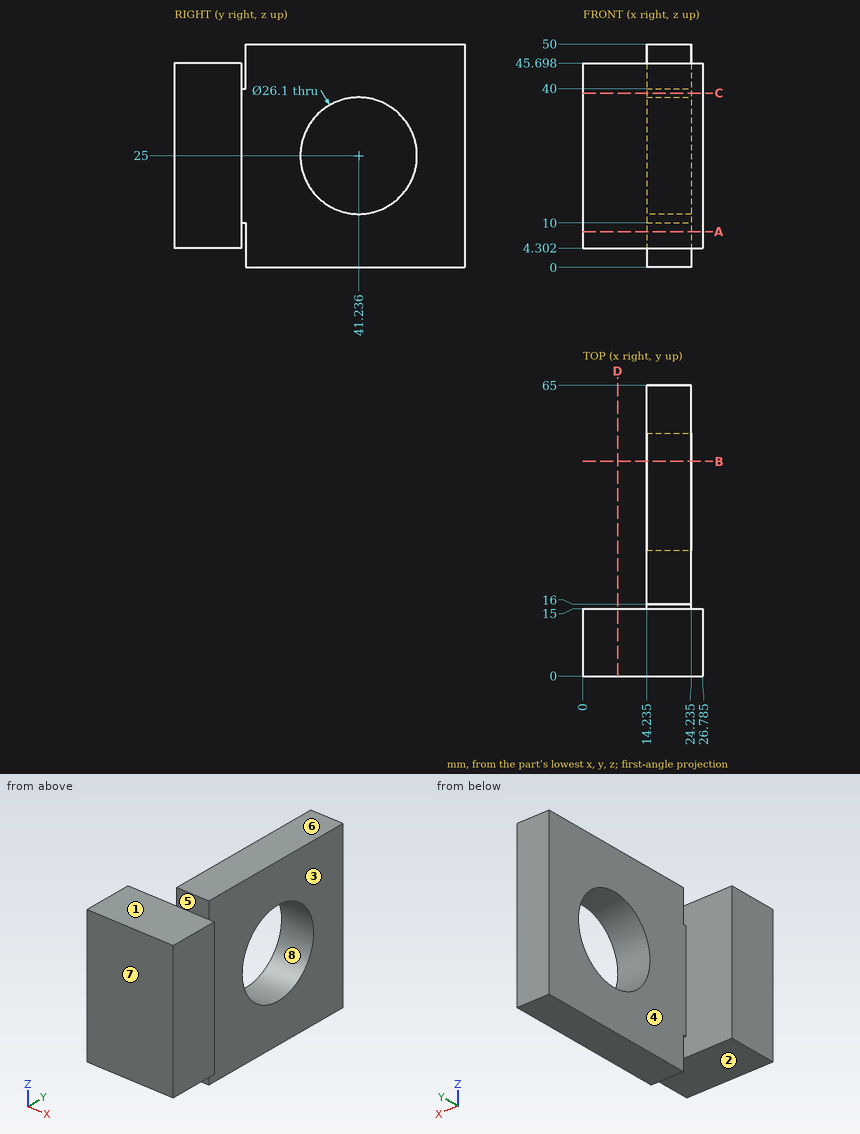
Design review of the part shown in the three views and the two pictorial views. Dimensions are in mm from the part's minimum x, y and z. A direction names the side the tool comes from. Round coordinates to 2 decimals unless told otherwise and drop trailing zeros. Write each loop counter-clockwise with the first axis right and the second up, starting at its lowest first coordinate (ties: lowest second). Pieces come first, ordered by that corner, then holes. Notation, with made-up numbers: (80, -3) - (132, -3) arc R21 cw to (132, 22) - close; hole circle Ø8 at (64, 82.25). An arc over 180 degrees is marked (long way). Return JSON: item names as keys, results as strings. Group by question number.
Item 1: We need section D-D on x = 7.75. Write out the cut boundary in (y, z), and give its area (3 significant figures).
Item 2: The part is to be moulded in two halves that separate along Y. For the marked faces 6, 7 and 8, say which applies: pulls with the +Y half, pulls with the -Y half, needs draft (parallel to the pull), parting line crosses it, or undercut.
Item 3: We need section C-C on z = 39. Write out the cut boundary in (x, y) (1 decimal), and give its area (3 significant figures).
Item 4: We need section B-B on y = 48. Write out the cut boundary in (x, z) (1 decimal), and give its area (3 significant figures).
Item 5: Insertion check: P1, Ø3, axis at y = 43.5, z = 41, coming from the -X side (1 decimal); P2, Ø12, axis at x = 13.5, y = 5.5, coming from the +Z side; P3, Ø3, axis at y = 23, z = 19, coming from the +X side (1 decimal); P4, Ø23.5, axis at y = 41.24, z = 25, coming from the -X side. Each pin has a flat end and moves straight along its axis. Give the tip position at first contact, or say it passes through.
Item 6: For probe 1 along Y at (x, z) = (21.5, 25); probe 2 along Y at (x, z) = (19, 5); probe 3 along Z at (x, y) = (10.75, 5), list the stretches that pass through material, from the lowest coordinate up. Write a range as [from, to].
Item 7: We need section A-A on z = 8. Write out the cut boundary in (x, y) (1 decimal), and give its area (3 significant figures).
Item 8: Machinability: for the marked faces 1, 2, 3, 4 and 5, which of the approach directions +Z, -Z, +X, -X, +Y, -Y give a long, thin tool a straight path to every point of the face, cutting with its end or side? Answer none if there is none.
Model answer:
{
 "1": {"outline": "(0, 4.3) - (15, 4.3) - (15, 45.7) - (0, 45.7) - close", "area": "621 mm²"},
 "2": {"face 6": "needs draft", "face 7": "pulls with the -Y half", "face 8": "undercut"},
 "3": {"outline": "(0, 0) - (26.8, 0) - (26.8, 15) - (24.2, 15) - (24.2, 65) - (14.2, 65) - (14.2, 15) - (0, 15) - close", "area": "902 mm²"},
 "4": {"outline": "(14.2, 0) - (24.2, 0) - (24.2, 13.8) - (14.2, 13.8) - close; (14.2, 36.2) - (24.2, 36.2) - (24.2, 50) - (14.2, 50) - close", "area": "277 mm²"},
 "5": {"P1": "stops at x = 14.2", "P2": "stops at z = 45.7", "P3": "stops at x = 24.2", "P4": "passes through"},
 "6": {"probe 1": "y = [0, 28.19], [54.29, 65]", "probe 2": "y = [0, 15], [16, 65]", "probe 3": "z = [4.3, 45.7]"},
 "7": {"outline": "(0, 0) - (26.8, 0) - (26.8, 15) - (0, 15) - close; (14.2, 16) - (24.2, 16) - (24.2, 65) - (14.2, 65) - close", "area": "892 mm²"},
 "8": {"face 1": "+Z, +X, -X, -Y", "face 2": "-Z, +X, -X, -Y", "face 3": "+Z, -Z, +X, +Y", "face 4": "+Z, -Z, -X, +Y", "face 5": "+Z, +X, -X"}
}
